Autodesk Inventor part; units mm, degrees
ref_plane "YZ Plane" through (0, 0, 0) normal (1, 0, 0) x (0, 1, 0)
ref_plane "XZ Plane" through (0, 0, 0) normal (0, 1, 0) x (-1, 0, 0)
ref_plane "XY Plane" through (0, 0, 0) normal (0, 0, 1) x (1, 0, 0)
sketch "Sketch1" plane through (0, 0, 0) normal (0, 0, 1) x (1, 0, 0)
  line L0 (6, 12) -> (4, 12)
  line L1 (6, 12) -> (8, 12)
  line L2 (12, 6) -> (12, 8)
  line L3 (12, 6) -> (12, 4)
  line L4 (0, 6) -> (0, 8)
  line L5 (0, 6) -> (0, 4)
  line L6 (6, 0) -> (8, 0)
  line L7 (6, 0) -> (4, 0)
  line L8 (4, 0) -> (4, 4)
  line L9 (4, 4) -> (0, 4)
  line L10 (0, 8) -> (4, 8)
  line L11 (4, 8) -> (4, 12)
  line L12 (8, 12) -> (8, 8)
  line L13 (8, 8) -> (12, 8)
  line L14 (8, 0) -> (8, 4)
  line L15 (8, 4) -> (12, 4)
  point P0 (0, 0)
  dimension "d2" = 2
  dimension "d3" = 2
  dimension "d4" = 2
  dimension "d5" = 2
  dimension "d6" = 2
  dimension "d7" = 2
  dimension "d8" = 2
  dimension "d9" = 2
extrude "Extrusion1" add sketch "Sketch1" along normal blind 5
sketch "Sketch2" plane through (0, 0, 5) normal (0, 0, 1) x (1, 0, 0)
  line L0 (0, 8) -> (0, 4)
  line L1 (0, 6) -> (12, 6)
  line L2 (12, 4) -> (12, 8)
  line L3 (8, 12) -> (4, 12)
  line L4 (6, 12) -> (6, 0)
  circle A0 centre (6, 6) radius 5
  point P0 (0, 0)
  dimension "d12" = 10
extrude "Extrusion2" add sketch "Sketch2" along normal blind 1
properties part number "PlusBtn"
Verification items for the finished model (mm, model axes). A direction names the side the tool comes from. Give positions to 0.01 mm unless a question says otherwise; leave off trailing zeros. Loops run counter-clockwise (first coordinate to the right, second up) from the corner with the lowest first, then second, coordinate; pieces in that order, holes last.
1) Thickness scan on line 1 along Z through (x, y) = (3.5, 8.5); line 2 along Z through (x, y) = (6.75, 11.25); line 3 along X through (y, z) = (11, 4.45). Record the ranges inside material, lowest first.
2) Depth check by flat-ended pin: pin 1 Ø2 at (y, z) = (2, 2.5) entering from +X; pin 2 Ø3 at (x, z) = (2, 2) entering from +Y; pin 3 Ø0.8 at (x, y) = (10, 9.5) entering from -Z; pin 4 Ø0.8 at (x, y) = (2, 10) entering from -Z. Enter the tip coordinate at first touch or a pass-through.
3) Draft check along Z on faces 4 (the flat face through (0.5, 6, 5)), 5 (the flat face through (4, 10, 2)), 6 (the flat face through (9, 9, 5)). Enter one of: pulls with the +Z half, pulls with the -Z half, needs draft (parallel to the pull), parting line crosses it, or undercut.
4) Sectioned sample at B-B, the plane z = 2.1. Enter the section's corners in (x, y).
5) Set-up check for faces 1 (the flat face through (4, 2, 2)), 2 (the flat face through (8, 2, 2)), 3 (the flat face through (2, 8, 2)): record each of +Z, -Z, +X, -X, +Y, -Y from which the full face is reachable in a straight line by a thin tool's end or side.
6) Sectioned sample at A-A, the plane y = 6. Enter the section's corners in (x, z), then the cut area to 3 significant figures.
Answers:
1. line 1: z = 5 to 6
1. line 2: z = 0 to 5
1. line 3: x = 4 to 8
2. pin 1: stops at x = 8
2. pin 2: stops at y = 8
2. pin 3: stops at z = 5
2. pin 4: passes through
3. face 4: pulls with the +Z half
3. face 5: needs draft
3. face 6: pulls with the -Z half
4. outline: (0, 4) - (4, 4) - (4, 0) - (8, 0) - (8, 4) - (12, 4) - (12, 8) - (8, 8) - (8, 12) - (4, 12) - (4, 8) - (0, 8) - close
5. face 1: -Z, -X, -Y
5. face 2: -Z, +X, -Y
5. face 3: -Z, -X, +Y
6. outline: (0, 0) - (12, 0) - (12, 5) - (11, 5) - (11, 6) - (1, 6) - (1, 5) - (0, 5) - close
6. area: 70.0 mm2
